Read the model definition and answer for the solid it produces. Units are mm, in the model's axes. A direction names the side the tool comes from. Coordinates: 2 decimals unless noted, no trailing zeros. Loops run counter-clockwise (first coordinate to the right, second up) from the corner with the lowest first, then second, coordinate; pieces in that order, holes last. Notation, with made-up numbers: M 61,79.25 L 100,79.25 A31 ccw 100,112.25 Z; hole C -24.5,24 d10. An arc over 180 degrees is marked long. Put each result on its own line as item: value.
from build123d import *

# Parameters (mm, degrees)
F1_DEPTH  = 55
F2_R      = 17.5
F3_R      = 39
F4_DEPTH  = 10
F5_R      = 32.5
F6_DEPTH  = 210
F8_DEPTH  = 45
F10_DEPTH = 25
F11_R     = 25
F16_DEPTH = 30
F17_R     = 20


with BuildPart() as f1:
    # F0 (on Top) → F1 (new body)
    with BuildSketch(Plane.XY):
        with BuildLine():
            Line((-17.5, 275), (-19, 35.1994318136))
            ThreePointArc((-19, 35.1994318136), (-23.5114100917, 32.360679775), (-27.6053261031, 28.9472964324))
            Line((-27.6053261031, 28.9472964324), (-256.1327445796, 101.6231624883))
            Line((-256.1327445796, 101.6231624883), (-266.9483393827, 68.3361844179))
            Line((-266.9483393827, 68.3361844179), (-39.3479718893, -7.1928511869))
            ThreePointArc((-39.3479718893, -7.1928511869), (-38.0422606518, -12.360679775), (-36.0610298022, -17.309018736))
            Line((-36.0610298022, -17.309018736), (-175.798741782, -212.193431538))
            Line((-175.798741782, -212.193431538), (-147.4831469789, -232.7659153682))
            Line((-147.4831469789, -232.7659153682), (-5.318384016, -39.6448583231))
            ThreePointArc((-5.318384016, -39.6448583231), (0, -40), (5.318384016, -39.6448583231))
            Line((5.318384016, -39.6448583231), (147.4831469789, -232.7659153682))
            Line((147.4831469789, -232.7659153682), (175.798741782, -212.193431538))
            Line((175.798741782, -212.193431538), (36.0610298022, -17.309018736))
            ThreePointArc((36.0610298022, -17.309018736), (38.0422606518, -12.360679775), (39.3479718893, -7.1928511869))
            Line((39.3479718893, -7.1928511869), (266.9483393827, 68.3361844179))
            Line((266.9483393827, 68.3361844179), (256.1327445796, 101.6231624883))
            Line((256.1327445796, 101.6231624883), (27.6053261031, 28.9472964324))
            ThreePointArc((27.6053261031, 28.9472964324), (23.5114100917, 32.360679775), (19, 35.1994318136))
            Line((19, 35.1994318136), (17.5, 275))
            Line((17.5, 275), (-17.5, 275))
        make_face()
    extrude(amount=F1_DEPTH)

    # F2
    f2_edges = [f1.edges().sort_by_distance(p)[0] for p in [
        (17.5, 275, 27.5),
        (256.132745, 101.623162, 27.5),
        (266.948339, 68.336184, 27.5),
        (-17.5, 275, 27.5),
        (-256.132745, 101.623162, 27.5),
        (-266.948339, 68.336184, 27.5),
        (-175.798742, -212.193432, 27.5),
        (-147.483147, -232.765915, 27.5),
        (147.483147, -232.765915, 27.5),
        (175.798742, -212.193432, 27.5),
    ]]
    fillet(f2_edges, radius=F2_R)

    # F3 (on face) → F4 (join)
    with BuildSketch(Plane(origin=(0, 0, 0), x_dir=(1, 0, 0), z_dir=(0, 0, -1))):
        Circle(F3_R)
    extrude(amount=F4_DEPTH)

    # F5 (on face) → F6 (join)
    with BuildSketch(Plane(origin=(0, 0, -10), x_dir=(1, 0, 0), z_dir=(0, 0, -1))):
        Circle(F5_R)
    extrude(amount=F6_DEPTH)

    # F7 (on face) → F8 (join)
    with BuildSketch(Plane(origin=(0, 0, -220), x_dir=(1, 0, 0), z_dir=(0, 0, -1))):
        with BuildLine():
            Line((95, 190), (-95, 190))
            ThreePointArc((-95, 190), (-165.7106781187, 160.7106781187), (-195, 90))
            Line((-195, 90), (-195, -10))
            ThreePointArc((-195, -10), (-142.2792206136, -137.2792206136), (-15, -190))
            Line((-15, -190), (15, -190))
            ThreePointArc((15, -190), (142.2792206136, -137.2792206136), (195, -10))
            Line((195, -10), (195, 90))
            ThreePointArc((195, 90), (165.7106781187, 160.7106781187), (95, 190))
        make_face()
    extrude(amount=F8_DEPTH)

    # F9 (on face) → F10 (join)
    with BuildSketch(Plane(origin=(0, 0, -265), x_dir=(1, 0, 0), z_dir=(0, 0, -1))):
        with BuildLine():
            Line((95, 190), (-95, 190))
            ThreePointArc((-95, 190), (-165.7106781187, 160.7106781187), (-195, 90))
            Line((-195, 90), (-195, -10))
            ThreePointArc((-195, -10), (-142.2792206136, -137.2792206136), (-15, -190))
            Line((-15, -190), (15, -190))
            ThreePointArc((15, -190), (142.2792206136, -137.2792206136), (195, -10))
            Line((195, -10), (195, 90))
            ThreePointArc((195, 90), (165.7106781187, 160.7106781187), (95, 190))
        make_face()
    extrude(amount=F10_DEPTH)

    # F11
    f11_edges = [f1.edges().sort_by_distance(p)[0] for p in [
        (195, -40, -290),
    ]]
    fillet(f11_edges, radius=F11_R)

    # F14: sweep along a path in F13
    with BuildLine(Plane.YZ) as f14_path:
        Line((190, -242.5), (225, -242.5))
        ThreePointArc((225, -242.5), (260.3553390593, -257.1446609407), (275, -292.5))
        Line((275, -292.5), (275, -462.5))
    # F12 (on face) → F14 (sweep)
    with BuildSketch(Plane(origin=(0, 190, 0), x_dir=(-1, 0, 0), z_dir=(0, 1, 0))):
        with BuildLine():
            Line((17.5, -227.5), (-17.5, -227.5))
            ThreePointArc((-17.5, -227.5), (-28.1066017178, -231.8933982822), (-32.5, -242.5))
            ThreePointArc((-32.5, -242.5), (-28.1066017178, -253.1066017178), (-17.5, -257.5))
            Line((-17.5, -257.5), (17.5, -257.5))
            ThreePointArc((17.5, -257.5), (28.1066017178, -253.1066017178), (32.5, -242.5))
            ThreePointArc((32.5, -242.5), (28.1066017178, -231.8933982822), (17.5, -227.5))
        make_face()
    sweep(path=f14_path.line)

    # F15 (on face) → F16 (join)
    with BuildSketch(Plane.XZ.offset(-260)):
        with BuildLine():
            Line((107.5, -372.5), (-107.5, -372.5))
            ThreePointArc((-107.5, -372.5), (-160.533008589, -394.466991411), (-182.5, -447.5))
            Line((-182.5, -447.5), (-182.5, -477.5))
            ThreePointArc((-182.5, -477.5), (-160.533008589, -530.533008589), (-107.5, -552.5))
            Line((-107.5, -552.5), (107.5, -552.5))
            ThreePointArc((107.5, -552.5), (160.533008589, -530.533008589), (182.5, -477.5))
            Line((182.5, -477.5), (182.5, -447.5))
            ThreePointArc((182.5, -447.5), (160.533008589, -394.466991411), (107.5, -372.5))
        make_face()
    extrude(amount=F16_DEPTH)

    # F17
    f17_edges = [f1.edges().sort_by_distance(p)[0] for p in [
        (-160.533009, 230, -530.533009),
    ]]
    fillet(f17_edges, radius=F17_R)


solid = f1.part
1) Find section B-B, the plane z = -179.5. Write down the section's boundary in (x, y), plus the area to 3 significant figures.
Answer list:
outline: C 0,0 d65
area: 3,320 mm^2
2) Given pin 1 Ø8 at (x, z) = (94.5, -459) entering from +Y; pin 2 Ø3 at (x, z) = (101, -241.5) entering from +Y; pin 3 Ø5 at (x, z) = (20.5, -243.5) entering from -Y, each flat-ended and moving along its own axis, determine where each tip first touches the part or whether it passes through.
Answer list:
pin 1: stops at y = 260
pin 2: stops at y = 168.93
pin 3: stops at y = -190
3) Find section A-A, the plane y = 199. Write down the section's boundary in (x, z).
Answer list:
outline: M -17.98,0 L 17.98,0 L 17.98,55 L -17.98,55 Z; M -17.5,-257.5 L 17.5,-257.5 A15 ccw 17.5,-227.5 L -17.5,-227.5 A15 ccw Z
4) Determine the mould class of faces 6 (the cylindrical face through (32.496, 275.33, -378.69)), 7 (the flat face through (0, 290, -379)), 8 (the cylindrical face through (-1.505, 235.703, -378.514)) for opening direction Y: released by +Y, released by -Y, zero draft, split by the parting line, or undercut.
Answer list:
face 6: undercut
face 7: released by +Y
face 8: released by -Y
5) Find section C-C, the plane x = -153. Count the separate pieces of the cut face and the enclosed holes in it, plus the area to 3 significant figures.
Answer list:
separate pieces: 4
enclosed holes: 0
area: 29,300 mm^2
6) Straight lines are drawn through the part: line 1 (Z direction, x = 96.5, y = -120); line 2 (Y direction, x = -160, z = -424); line 3 (Y direction, x = 16.5, z = -305). For each, find the intervals that lie inside material, in ascending order. Write a range as [from, to].
Answer list:
line 1: z = [-290, -220], [0, 55]
line 2: y = [230.16, 260]
line 3: y = [260, 290]
7) Which of the six approach directions +Z, -Z, +X, -X, +Y, -Y give full straight-line access (tool end or side, diameter ignored) to faces 1 (the cylindrical face through (31, -9.76, -113.53)), 2 (the flat face through (70.323, -127.949, 27.115)), 3 (the flat face through (135.066, 63.122, 27.115)), 4 (the cylindrical face through (-0.245, 249.475, -267.481)), 5 (the flat face through (-2, -2, -290))?
Answer list:
face 1: none
face 2: +Z, -Y
face 3: +Z, +Y
face 4: +X, -X
face 5: -Z, +X, -X, -Y
